Input: part model. Units: mm. Frame: model coordinates. A direction names the side the tool comes from. Coordinates: 2 decimals unless noted, no trailing zeros. Write each loop counter-clockwise with the first axis right and the second up, starting at its lowest first coordinate (ties: lowest second). Pieces come first, ordered by that corner, then holes. Notation, with made-up numbers: (27, 1) - (82, 1) arc R15 cw to (82, 28) - close; hole circle Ø2 at (23.25, 25.25). An arc over 180 degrees is marked (long way). Use a Markdown table: item, result. Add a question column.
Q1. Set-up query: faces 1 (the face through (40, 10, -15)), 2 (the face through (64.297, 5.07, -33.986)), 3 (the face through (30, 20, -35)). Return all of +Z, -Z, +X, -X, +Y, -Y with unobstructed straight access to the full face (end or side cutting, diameter ignored); none if empty.
Q2. Section query B-B (x = 17). Return the cut outline in (y, z).
Q3. Material intervals for probe 1 along Z at (x, y) = (50, 6.25); probe 2 along X at (y, z) = (5, -20); probe 3 along Y at (x, z) = (53.5, -4.5), sorted ascending. Write a range as from..to.
Q4. Pin query (flat end, axial travel): P1, Ø3, axis at y = 3.5, z = -31.5, coming from the +X side; P2, Ø1, axis at x = 30, z = -12, coming from the +Y side; P3, Ø3, axis at y = 21.5, z = -31, coming from the +X side. Return the tip coordinate at first contact, or that it passes through.
Q5. Section query D-D (y = 12). Return the cut outline in (x, z), then the cut area to 3 significant figures.
Q6. Mould query, pull axis X, two halves, no side actions, for faces 4 (the face through (58.872, 4.93, -15.386)), 5 (the face through (0, 15, -20)), 6 (the face through (11.46, 26.18, -18.54)). Classes: released by +X, released by -X, zero draft, split by the parting line, or undercut.
Q7. Section query C-C (x = 53). Return the cut outline in (y, z).
Autodesk Inventor part; units mm, degrees
ref_plane "YZ Plane" through (0, 0, 0) normal (1, 0, 0) x (0, 1, 0)
ref_plane "XZ Plane" through (0, 0, 0) normal (0, 1, 0) x (-1, 0, 0)
ref_plane "XY Plane" through (0, 0, 0) normal (0, 0, 1) x (1, 0, 0)
sketch "草圖1" plane through (0, 0, 0) normal (0, 1, 0) x (-1, 0, 0)
  line L0 (0, 0) -> (-70, 0)
  line L1 (-70, 0) -> (-70, -40)
  line L2 (-70, -40) -> (0, -40)
  line L3 (0, -40) -> (0, 0)
  dimension "d0" = 40
  dimension "d1" = 70
extrude "擠出1" add sketch "草圖1" along normal blind 10
sketch "草圖2" plane through (0, 10, 0) normal (0, 1, 0) x (1, 0, 0)
  line L0 (0, 0) -> (70, 0)
  line L1 (70, 40) -> (0, 40)
  line L2 (0, 0) -> (30, 0)
  line L3 (30, 0) -> (30, 40)
  line L4 (30, 40) -> (0, 40)
  line L5 (0, 40) -> (0, 0)
  dimension "d4" = 30
extrude "擠出2" add sketch "草圖2" along normal blind 20
sketch "草圖3" plane through (0, 30, 0) normal (0, 1, 0) x (1, 0, 0)
  line L0 (30, 30) -> (10, 0)
  line L1 (0, 0) -> (70, 0)
  line L2 (30, 0) -> (30, 30)
  line L3 (30, 0) -> (30, 40)
  line L4 (30, 0) -> (10, 0)
  dimension "d7" = 20
  dimension "d8" = 30
extrude "擠出3" cut sketch "草圖3" against normal blind 20
sketch "草圖4" plane through (0, 0, -40) normal (-1, 0, 0) x (0, 0, 1)
  line L0 (-20, 30) -> (40, 30)
  line L1 (10, 30) -> (40, 20)
  line L2 (40, 0) -> (40, 30)
  dimension "d11" = 10
  dimension "d12" = 30
extrude "擠出4" cut sketch "草圖4" against normal through all
fillet "圓角1" radius 20 2 edges at (70, 5, 0) (70, 5, -40)
hole "孔1" at (50, 10, -20) direction (0, -1, 0) diameter 20 depth 10 tip angle 118
properties part number "27"
Values follow:
| question | item | result |
|---|---|---|
| 1 | face 1 | +Z, +X, +Y |
| 1 | face 2 | -Z, +X, +Y, -Y |
| 1 | face 3 | +Z, -Z, +X, +Y |
| 2 | outline | (0, -40) - (30, -40) - (30, -30) - (23.5, -10.5) - (10, -10.5) - (10, 0) - (0, 0) - close |
| 3 | probe 1 | -40..-30, -10..0 |
| 3 | probe 2 | 0..40, 60..70 |
| 3 | probe 3 | 0..10 |
| 4 | P1 | x = 67.32 |
| 4 | P2 | y = 10 |
| 4 | P3 | x = 30 |
| 5 | outline | (0, -40) - (30, -40) - (30, -30) - (10, 0) - (0, 0) - close |
| 5 | area | 900 mm2 |
| 6 | face 4 | undercut |
| 6 | face 5 | released by -X |
| 6 | face 6 | zero draft |
| 7 | outline | (0, -39.77) - (10, -39.77) - (10, -29.54) - (0, -29.54) - close; (0, -10.46) - (10, -10.46) - (10, -0.23) - (0, -0.23) - close |
